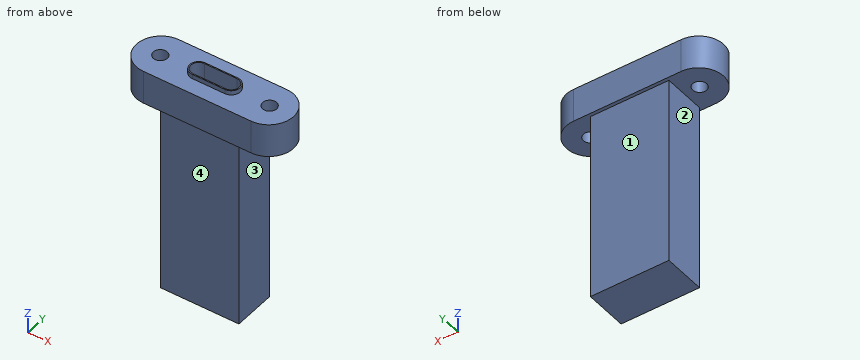
from build123d import *

# Parameters (mm, degrees)
SKETCH_1_W          = 14
SKETCH_1_H          = 7.6
EXTRUDE_1_DEPTH     = 34
EXTRUDE_2_DEPTH     = 6
EXTRUDE_3_DEPTH     = 0.8
CUT_EXTRUDE_1_DEPTH = 5
HOLE_WIZARD_M3_1_D  = 2.5


with BuildPart() as part:
    # 草图1 → 凸台-拉伸1 (new body)
    with BuildSketch(Plane.XY):
        Rectangle(SKETCH_1_W, SKETCH_1_H)
    extrude(amount=EXTRUDE_1_DEPTH)

    # 草图2 → 凸台-拉伸2 (add)
    with BuildSketch(Plane.XY.offset(34)):
        with BuildLine():
            Line((-9.6, 4.4), (9.6, 4.4))
            ThreePointArc((9.6, 4.4), (14, 0), (9.6, -4.4))
            Line((9.6, -4.4), (-9.6, -4.4))
            ThreePointArc((-9.6, -4.4), (-14, 0), (-9.6, 4.4))
        make_face()
    extrude(amount=EXTRUDE_2_DEPTH)

    # 草图3 → 凸台-拉伸3 (add)
    with BuildSketch(Plane.XY.offset(40)):
        with BuildLine():
            Line((-2.9, 1.6), (2.9, 1.6))
            ThreePointArc((2.9, 1.6), (4.5, 0), (2.9, -1.6))
            Line((2.9, -1.6), (-2.9, -1.6))
            ThreePointArc((-2.9, -1.6), (-4.5, 0), (-2.9, 1.6))
        make_face()
    extrude(amount=EXTRUDE_3_DEPTH)

    # 草图4 → 切除-拉伸1 (cut)
    with BuildSketch(Plane.XY.offset(40.8)):
        with BuildLine():
            Line((-2.9, -1.4), (2.9, -1.4))
            ThreePointArc((2.9, -1.4), (4.3, 0), (2.9, 1.4))
            Line((2.9, 1.4), (-2.9, 1.4))
            ThreePointArc((-2.9, 1.4), (-4.3, 0), (-2.9, -1.4))
        make_face()
    extrude(amount=-CUT_EXTRUDE_1_DEPTH, mode=Mode.SUBTRACT)

    # M3 螺纹孔1 (through all)
    with Locations(Plane.XY.offset(40)):
        with Locations((-9.75, 0), (9.75, 0)):
            Hole(HOLE_WIZARD_M3_1_D / 2)


solid = part.part
Here's how the part is built. I have some questions about the finished solid (model axes, mm). Face numbers are marked on the shaded views. A direction names the side the tool comes from. Coordinates: 2 decimals unless noted, no trailing zeros. Order: outer loops, then holes, each group sorted by start corner. A loop starts at its lowest first (then second) coordinate and runs counter-clockwise, first axis right, second up.
Item 1: If we section it at C-C on y = -2.5: List the corners of the cut face in (x, z) for me, plus the area to 3 significant figures.
Result sheet:
outline: (-13.22, 34) - (-7, 34) - (-7, 0) - (7, 0) - (7, 34) - (13.22, 34) - (13.22, 40) - (-13.22, 40) - close
area: 635 mm2
Item 2: For P1, Ø7, axis at x = 1.5, z = 18.5, coming from the -Y side; P2, Ø0.9, axis at x = -1, z = 40.5, coming from the +Y side; P3, Ø5, axis at x = 0.5, z = 5, coming from the +Y side; P4, Ø1.5, axis at x = 9.75, y = 0, coming from the -Z side, each with a flat end and sliding along its axis, tell me the tip position at first contact or that it passes through.
Result sheet:
P1: stops at y = -3.8
P2: stops at y = 1.6
P3: stops at y = 3.8
P4: passes through
Item 3: If we section it at B-B on x = 1: List the corners of the cut face in (y, z) for me, plus the area to 3 significant figures.
Result sheet:
outline: (-4.4, 34) - (-3.8, 34) - (-3.8, 0) - (3.8, 0) - (3.8, 34) - (4.4, 34) - (4.4, 40) - (1.6, 40) - (1.6, 40.8) - (1.4, 40.8) - (1.4, 35.8) - (-1.4, 35.8) - (-1.4, 40.8) - (-1.6, 40.8) - (-1.6, 40) - (-4.4, 40) - close
area: 300 mm2
Item 4: I need wall thicknesses on line 1 (Y direction, x = 1.5, z = 36); line 2 (Z direction, x = -6, y = 4.25); line 3 (X direction, y = 2, z = 8). Which ranges of each line are inside material? Lowest first, please.
Result sheet:
line 1: y = -4.4 to -1.4, 1.4 to 4.4
line 2: z = 34 to 40
line 3: x = -7 to 7
Item 5: If we section it at D-D on z = 16: List the corners of the cut face in (x, y) for me, plus the area to 3 significant figures.
Result sheet:
outline: (-7, -3.8) - (7, -3.8) - (7, 3.8) - (-7, 3.8) - close
area: 106 mm2
Item 6: For the marked faces 1, 2, 3 and 4, which set-ups out of +Z, -Z, +X, -X, +Y, -Y let a thin tool reach every point of the face, with its end or its side?
Result sheet:
face 1: -Z, +X, -X, +Y
face 2: -Z, -X, +Y, -Y
face 3: -Z, +X, +Y, -Y
face 4: -Z, +X, -X, -Y
Item 7: If we section it at A-A on y = 0: List the corners of the cut face in (x, z) for me, plus the area to 3 significant figures.
Result sheet:
outline: (-14, 34) - (-11, 34) - (-11, 40) - (-14, 40) - close; (-8.5, 34) - (-7, 34) - (-7, 0) - (7, 0) - (7, 34) - (8.5, 34) - (8.5, 40) - (4.5, 40) - (4.5, 40.8) - (4.3, 40.8) - (4.3, 35.8) - (-4.3, 35.8) - (-4.3, 40.8) - (-4.5, 40.8) - (-4.5, 40) - (-8.5, 40) - close; (11, 34) - (14, 34) - (14, 40) - (11, 40) - close
area: 578 mm2
